Part model, mm, in its own coordinate system. Face numbers are marked on the shaded views. A direction names the side the tool comes from. Coordinates: 2 decimals unless noted, no trailing zeros. Loops run counter-clockwise (first coordinate to the right, second up) from the corner with the lowest first, then second, coordinate; pieces in that order, holes last. Notation, with made-up numbers: (-11, 10.25) - (47, 10.25) arc R30 cw to (47, 34.25) - close; hole circle Ø5 at (67.5, 8). An arc over 180 degrees is marked (long way). Use a Markdown table: item, result. Add a question column.
1. 3-axis set-ups, long thin cutter, end or side, ignore diameter. For the marked faces 5, 6 and 7: which of +Z, -Z, +X, -X, +Y, -Y reach the whole face in a straight line?
2. Band-saw the part on C-C, the plane y = -27.5. Give the cut face in (x, z).
3. Wall check: probe 1 along X at (y, z) = (24, 0); probe 2 along Y at (x, z) = (-98.5, -22.5); probe 3 along Z at (x, y) = (-17, 27). Give the ranges that are in metal, low to high. Write a range as [from, to].
4. Drop flat-ended pins along their axis: pin 1 (3 mm diameter, centred on x = -83, z = -88, fed in from -Y); pin 2 (4 mm diameter, centred on y = -37.5, z = 68, fed in from -X); pin 3 (3 mm diameter, centred on y = -30, z = 11.5, fed in from +X). Give the stop position or say it passes through.
5. Band-saw the part on D-D, the plane x = -89. Give the cut face in (y, z), plus the area to 3 significant figures.
6. Pull direction X, two halves, no side cores. Call the marked faces 1, 2, 3 and 4: pulls with the +X half, pulls with the -X half, needs draft (parallel to the pull), parting line crosses it, or undercut.
from build123d import *


with BuildPart() as f1:
    # F0 (on Right) → F1 (revolve)
    with BuildSketch(Plane.YZ):
        Polygon((20, 100), (0, 100), (-20, 100), (-20, 125), (-37.5, 125), (-37.5, 82.5), (-20, 82.5), (-20, 37.5), (-50, 37.5), (-50, 12.5), (0, 12.5), (50, 12.5), (50, 37.5), (20, 37.5), (20, 82.5), (37.5, 82.5), (37.5, 125), (20, 125), align=None)
    revolve(axis=Axis((0, -3.476026, 0), (0, 1, 0)))


solid = f1.part
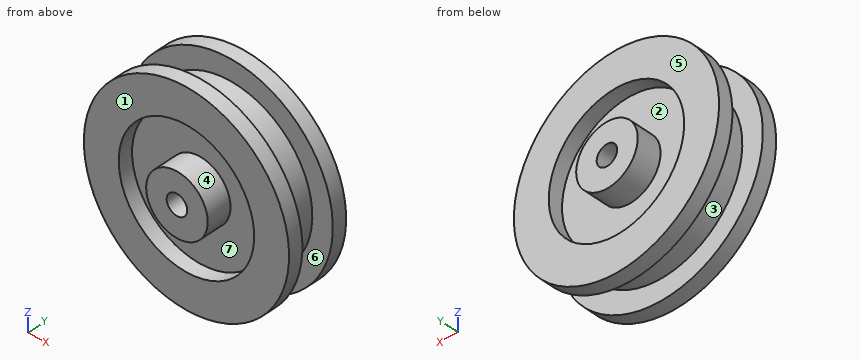
Geometry check:
| question | item | result |
|---|---|---|
| 1 | face 5 | +Y |
| 1 | face 6 | none |
| 1 | face 7 | -Y |
| 2 | outline | circle Ø250 at (0, 0); circle Ø75 at (0, 0); hole circle Ø165 at (0, 0); hole circle Ø25 at (0, 0) |
| 3 | probe 1 | x = [-125, -82.5], [-37.5, -12.5], [12.5, 37.5], [82.5, 125] |
| 3 | probe 2 | y = [-37.5, -20], [20, 37.5] |
| 3 | probe 3 | z = [-123.84, -80.73], [-33.43, 33.43], [80.73, 123.84] |
| 4 | pin 1 | stops at y = -37.5 |
| 4 | pin 2 | stops at x = -106.16 |
| 4 | pin 3 | stops at x = 124.6 |
| 5 | outline | (-37.5, -87.77) - (-20, -87.77) - (-20, -45.6) - (20, -45.6) - (20, -87.77) - (37.5, -87.77) - (37.5, 87.77) - (20, 87.77) - (20, 45.6) - (-20, 45.6) - (-20, 87.77) - (-37.5, 87.77) - close |
| 5 | area | 9,790 mm^2 |
| 6 | face 1 | needs draft |
| 6 | face 2 | undercut |
| 6 | face 3 | parting line crosses it |
| 6 | face 4 | undercut |
